For this review, take the finished solid that the model builds, in its own axes (mm). Face numbers are marked on the shaded views. A direction names the side the tool comes from. Give positions to 0.01 mm unless a question says otherwise; leave off trailing zeros. Write each loop counter-clockwise with the first axis right and the second up, starting at its lowest first coordinate (ties: lowest second). Pieces come first, ordered by that corner, then holes. Notation, with made-up numbers: M 46,-33 L 77,-33 A11 cw 77,-16 Z; hole C -29.5,44.5 d1. An arc over 180 degrees is marked long. Use one line per item in the form item = value. Start each with the question number.
Q1. Consider section C-C on z = -29. Write out the cut boundary in (x, y), and give its area (3 significant figures).
Q2. Consider section D-D on x = 23. Write out the cut boundary in (y, z).
Q3. For probe 1 along Y at (x, z) = (0, 3); probe 2 along Z at (x, y) = (28, -2); probe 3 along X at (y, z) = (0, -21), list the stretches that pass through material, from the lowest coordinate up. Write a range as [from, to].
Q4. Consider section A-A on y = 0. Write out the cut boundary in (x, z), and give its area (3 significant figures).
Q5. Clearance check with flat-ended pins moving along their axes: pin 1 Ø10 at (x, z) = (9.5, -19.5) entering from +Y; pin 2 Ø5 at (x, y) = (16, 8) entering from -Z; pin 3 Ø1 at (x, z) = (25.5, 3) entering from -Y; pin 4 Ø16 at (x, y) = (13.5, 5) entering from -Z. State where each tip first meets the part, or that it passes through.
Q6. Consider section B-B on z = 7.5. Write out the cut boundary in (x, y), and give its area (3 significant figures).
Q7. Tool access review of the marked faces 1 and 2: name each direction out of +Z, -Z, +X, -X, +Y, -Y from which nothing blocks a thin tool from reaching the whole face with its end or side.
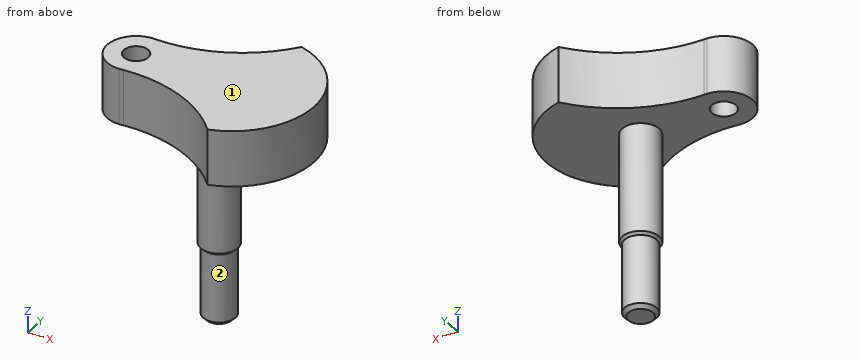
```python
from build123d import *

# Parameters (mm, degrees)
F0_R        = 2.5019
F1_DEPTH    = 11.43
F2_R        = 3.81
F3_DEPTH    = 23.0124
F4_R        = 3.2888740004
F5_DEPTH    = 14.5542
F6_S5_R     = 3.2888740004
F6_T6_DEPTH = 7
F7_SIZE     = 0.762


# Not quite as in the source:
# - a fillet or chamfer that OpenCascade refuses, or shapes differently, is made with other operations: its cross-section is extruded or revolved along the edge and cut away or added


with BuildPart() as f1:
    # F0 (on Top) → F1 (new body)
    with BuildSketch(Plane.XY):
        with BuildLine():
            ThreePointArc((23.9757987458, 16.602474899), (13.6238224038, 8.4064756981), (0.6664771358, 5.8677711678))
            ThreePointArc((0.6664771358, 5.8677711678), (4.4051566928, 3.9331316736), (5.9055, 0))
            ThreePointArc((5.9055, 0), (4.4601151914, -3.8706979641), (0.8314833277, -5.8466713372))
            ThreePointArc((0.8314833277, -5.8466713372), (13.3845311249, -8.052459978), (23.6582204203, -15.5953918211))
            ThreePointArc((23.6582204203, -15.5953918211), (35.9831697874, 0.3835426329), (23.9757987458, 16.602474899))
        make_face()
        with BuildLine():
            ThreePointArc((0.6664771358, 5.8677711678), (0.333126091, 5.8846486866), (0, 5.9055))
            ThreePointArc((0, 5.9055), (-5.9055, 0), (0, -5.9055))
            ThreePointArc((0, -5.9055), (0.4155226631, -5.8729903159), (0.8314833277, -5.8466713372))
            ThreePointArc((0.8314833277, -5.8466713372), (4.4601151914, -3.8706979641), (5.9055, 0))
            ThreePointArc((5.9055, 0), (4.4051566928, 3.9331316736), (0.6664771358, 5.8677711678))
        make_face()
        Circle(F0_R, mode=Mode.SUBTRACT)
        with BuildLine():
            ThreePointArc((0.6664771358, 5.8677711678), (0.3337720919, 5.8960602474), (0, 5.9055))
            ThreePointArc((0, 5.9055), (0.333126091, 5.8846486866), (0.6664771358, 5.8677711678))
        make_face()
        with BuildLine():
            ThreePointArc((0.8314833277, -5.8466713372), (0.4155226631, -5.8729903159), (0, -5.9055))
            ThreePointArc((0, -5.9055), (0.4167809184, -5.8907744751), (0.8314833277, -5.8466713372))
        make_face()
    extrude(amount=F1_DEPTH)

    # F2 (on face) → F3 (join)
    with BuildSketch(Plane(origin=(0, 0, 0), x_dir=(1, 0, 0), z_dir=(0, 0, -1))):
        with Locations((16.9372853817, 0)):
            Circle(F2_R)
    extrude(amount=F3_DEPTH)

    # F4 (on face) → F5 (join)
    with BuildSketch(Plane(origin=(0, 0, -23.0124), x_dir=(1, 0, 0), z_dir=(0, 0, -1))):
        with Locations((16.9372853817, 0)):
            Circle(F4_R)
    extrude(amount=F5_DEPTH)

    # F6: chamfer of 0.762 on 1 edges, made by hand


with BuildPart() as f6_tool2:
    # F6_s3 → F6_t4 (revolve)
    with BuildSketch(Plane.XZ):
        Polygon((20.7472853817, -22.2504), (19.9852853817, -23.0124), (20.7472853817, -23.0124), align=None)
    revolve(axis=Axis((16.9372853817, 0, -23.0124), (0, 0, -1)))

    # F6_s5 → F6_t6 (cut, symmetric)
    with BuildSketch(Plane.XY.offset(-22.6)):
        with Locations((16.9372853817, 0)):
            Circle(F6_S5_R)
    extrude(amount=F6_T6_DEPTH, both=True, mode=Mode.SUBTRACT)


with BuildPart() as f1_1:
    add(f1.part)

    # F6_t1: cut F6_tool2
    add(f6_tool2.part, mode=Mode.SUBTRACT)

    # F7
    f7_edges = [f1_1.edges().sort_by_distance(p)[0] for p in [
        (13.648411, 0, -37.5666),
    ]]
    chamfer(f7_edges, length=F7_SIZE)


solid = f1_1.part
```
Working result:
q1.outline = C 16.94,0 d6.58
q1.area = 34.0 mm²
q2.outline = M -14.85,0 L 15.42,0 L 15.42,11.43 L -14.85,11.43 Z
q3.probe_1 = [-5.91, -2.5], [2.5, 5.91]
q3.probe_2 = [0, 11.43]
q3.probe_3 = [13.13, 20.75]
q4.outline = M -5.91,0 L -2.5,0 L -2.5,11.43 L -5.91,11.43 Z; M 2.5,0 L 13.13,0 L 13.13,-22.25 L 13.65,-22.77 L 13.65,-36.8 L 14.41,-37.57 L 19.46,-37.57 L 20.23,-36.8 L 20.23,-22.77 L 20.75,-22.25 L 20.75,0 L 35.97,0 L 35.97,11.43 L 2.5,11.43 Z
q4.area = 691 mm²
q5.pin_1 = 2.93
q5.pin_2 = 0
q5.pin_3 = -15.17
q5.pin_4 = -37.57
q6.outline = M 0.67,5.87 A5.91 ccw long 0.83,-5.85 A27.99 cw 23.66,-15.6 A16.74 ccw 23.98,16.6 A27.99 cw Z; hole C 0,0 d5
q6.area = 737 mm²
q7.face_1 = +Z, +X, -X, +Y, -Y
q7.face_2 = -Z
